from build123d import *

# Parameters (mm, degrees)
F0_W        = 254
F0_H        = 203.2
F1_DEPTH    = 3.175
F2_T1_DEPTH = 511.175
F3_R        = 3.175
F4_DEPTH    = 3.175


# Not quite as in the source:
# - a fillet or chamfer that OpenCascade refuses, or shapes differently, is made with other operations: its cross-section is extruded or revolved along the edge and cut away or added


with BuildPart() as f1:
    # F0 (on Top) → F1 (new body)
    with BuildSketch(Plane.XY):
        with Locations((-9.1833584011, 11.7048747692)):
            Rectangle(F0_W, F0_H)
    extrude(amount=F1_DEPTH)

    # F2: fillet of radius 101.6 on 2 edges, made by hand

    # F2_s2 → F2_t1 (cut)
    with BuildSketch(Plane.XY.offset(-254)):
        with BuildLine():
            add(Edge.make_bspline(
                [(-136.1833584011, 11.7048747692), (-136.1833584011, 113.3048747692), (-34.5833584011, 113.3048747692)],
                knots=[0, 0, 0, 1, 1, 1], degree=2, weights=[1, 1, 1]))
            Line((-34.5833584011, 113.3048747692), (-136.1833584011, 113.3048747692))
            Line((-136.1833584011, 113.3048747692), (-136.1833584011, 11.7048747692))
        make_face()
        with BuildLine():
            add(Edge.make_bspline(
                [(117.8166415989, 11.7048747692), (117.8166415989, 113.3048747692), (16.2166415989, 113.3048747692)],
                knots=[0, 0, 0, 1, 1, 1], degree=2, weights=[1, 1, 1]))
            Line((16.2166415989, 113.3048747692), (117.8166415989, 113.3048747692))
            Line((117.8166415989, 113.3048747692), (117.8166415989, 11.7048747692))
        make_face()
    extrude(amount=F2_T1_DEPTH, mode=Mode.SUBTRACT)

    # F3 (on face) → F4 (cut)
    with BuildSketch(Plane.XY.offset(3.175)):
        with Locations((-85.3833584011, -77.1951252308)):
            Circle(F3_R)
        with Locations((67.0166415989, -77.1951252308)):
            Circle(F3_R)
    extrude(amount=-F4_DEPTH, mode=Mode.SUBTRACT)


solid = f1.part
Input: part model. Units: mm. Frame: model coordinates. Coordinates: 2 decimals unless noted, no trailing zeros. Write each question's results on one line, items separated by ' | '. Start each with the question number.
Q1. Pin query (flat end, axial travel): pin 1 (1.5 mm diameter, centred on x = 54, z = 2.5, fed in from +Y). Return the tip coordinate at first contact, or that it passes through.
Q2. Pull-direction query (Y, two-part tool) for faces 1 (the flat face through (-11, 13, 0)), 2 (the cylindrical face through (-88.555, -77.056, 1.61)); classes: released by +Y, released by -Y, zero draft, split by the parting line, or undercut.
Q3. Section A-A, the plane z = 1.6. State how many separate pieces and enclosed holes the cut face has, plus the area to 3 significant figures.
Q4. Ray query, line 1 (Y direction, x = 69.5, z = 1); line 2 (Y direction, x = 89, z = 2.75); line 3 (Y direction, x = 95, z = 2.7). Return the intervals inside material, ascending. Write a range as from..to.
Found:
1) pin 1: y = 109.13
2) face 1: zero draft | face 2: undercut
3) separate pieces: 1 | enclosed holes: 2 | area: 48,100 mm2
4) line 1: -89.9..-79.17, -75.22..103.52 | line 2: -89.9..91.11 | line 3: -89.9..85.18
